Read the model definition and answer for the solid it produces. Units are mm, in the model's axes. Face numbers are marked on the shaded views. A direction names the side the tool comes from. Round coordinates to 2 decimals unless told otherwise and drop trailing zeros. Order: outer loops, then holes, each group sorted by start corner. A loop starts at its lowest first (then second) coordinate and runs counter-clockwise, first axis right, second up. Notation, with made-up numbers: (-21.75, 81.5) - (-13.75, 81.5) arc R8 cw to (-13.75, 95.5) - close; hole circle Ø2 at (-34.75, 36). An arc over 180 degrees is marked (long way). Answer as a JSON object with one key per item and string values. Group by question number.
Q1. A tool of negligible diameter and unlimited length cuts with its end or side. For the marked faces 4, 5 and 6, from which of +Z, -Z, +X, -X, +Y, -Y can it reach the whole face along a straight path? Write none if from no direction.
Q2. A cutting plane is placed at B-B on x = 2.54. Determine the outline of the cut face in (y, z).
Q3. Consider line 1 (X direction, y = -1.25, z = 2.75); line 2 (X direction, y = 8, z = 3.5); line 3 (X direction, y = 0, z = 2). Determine where each line is inside the solid, lowest interval first.
Q4. The mould has two halves that part along Y. Classify the marked faces 1, 2 and 3: pulls with the +Y half, pulls with the -Y half, needs draft (parallel to the pull), parting line crosses it, or undercut.
Q5. A cutting plane is placed at A-A on y = 0. Count the separate pieces of the cut face and the enclosed holes in it, and give its area (3 significant figures).
Q6. Given pin 1 Ø8 at (x, y) = (2.5, -10) entering from +Z; pin 2 Ø2 at (y, z) = (7, 1.5) entering from -X; pin 3 Ø2 at (x, z) = (-10.5, 6) entering from +Y, each flat-ended and moving along its own axis, determine where each tip first touches the part or whether it passes through.
Autodesk Inventor part; units mm, degrees
ref_plane "YZ Plane" through (0, 0, 0) normal (1, 0, 0) x (0, 1, 0)
ref_plane "XZ Plane" through (0, 0, 0) normal (0, 1, 0) x (-1, 0, 0)
ref_plane "XY Plane" through (0, 0, 0) normal (0, 0, 1) x (1, 0, 0)
sketch "Sketch1" plane through (0, 0, 0) normal (0, 0, 1) x (1, 0, 0)
  line L0 (0, 17.78) -> (0, -17.78)
  line L1 (-26.67, 0) -> (26.67, 0)
  line L2 (19.05, -12.7) -> (-19.05, -12.7)
  line L3 (-19.05, -12.7) -> (-19.05, 12.7)
  line L4 (-19.05, 12.7) -> (19.05, 12.7)
  line L5 (19.05, 12.7) -> (19.05, -12.7)
  line L6 (19.05, -12.7) -> (-19.05, 12.7) construction
  line L7 (-19.05, -12.7) -> (19.05, 12.7) construction
  point P0 (0, 0)
  dimension "d0" = 25.4
  dimension "d1" = 38.1
extrude "Extrusion1" add sketch "Sketch1" along normal blind 6.35
sketch "Sketch2" plane through (0, 0, 0) normal (0, 0, 1) x (1, 0, 0)
  line L0 (0, 4.445) -> (0, -4.445)
  line L1 (-14.986, 0) -> (5.461, 0)
  point P0 (0, 0)
  point P1 (2.54, 0)
  point P2 (-12.065, -3.175)
  dimension "d27" = 12.065
  dimension "d35" = 2.54
  dimension "d48" = 3.175
  dimension "d54" = 0
hole "Hole1" at (2.54, 0, 0) direction (0, 0, 1) diameter 4.1402 end through all
sketch "Sketch4" plane through (-19.05, 12.7, 6.35) normal (0, 1, 0) x (1, 0, 0)
  line L0 (19.05, 15.24) -> (19.05, -2.54)
  line L1 (45.72, 6.35) -> (-7.62, 6.35)
  line L2 (38.1, 6.35) -> (38.1, 0)
  line L3 (38.1, 0) -> (0, 0)
  point P0 (19.05, 6.35)
  point P1 (34.29, 3.175)
  point P2 (38.1, 12.7)
  dimension "d36" = 3.81
  dimension "d37" = 3.175
hole "Hole2" at (15.24, 12.7, 3.175) direction (0, -1, 0) diameter 3.175 end through all
hole "Hole3" at (-12.065, -3.175, 0) direction (0, 0, 1) diameter 8.636 end through all counterbore diameter 9.525 counterbore depth 0.635
sketch "Sketch5" plane through (0, 0, 6.35) normal (0, 0, 1) x (1, 0, 0)
  line L0 (19.05, -12.7) -> (19.05, 12.7)
  line L1 (19.05, 12.7) -> (-19.05, 12.7)
  line L2 (-19.05, -12.7) -> (19.05, -12.7)
  line L3 (19.05, 12.7) -> (12.065, 12.7)
  line L4 (12.065, 12.7) -> (12.065, -12.7)
  line L5 (12.065, -12.7) -> (19.05, -12.7)
  line L6 (19.05, -12.7) -> (19.05, 12.7)
  circle A0 centre (2.54, 0) radius 2.0701
  point P0 (0, 0)
  dimension "d39" = 6.985
  dimension "d40" = 9.525
extrude "Extrusion3" add sketch "Sketch5" along normal blind 1.27 contours L2 L4 L1 L0
sketch "Sketch6" plane through (0, 0, 0) normal (0, 0, 1) x (1, 0, 0)
  line L0 (0, 13.335) -> (0, -13.335)
  line L1 (-26.67, 0) -> (26.67, 0)
  line L2 (12.065, 12.7) -> (-19.05, 12.7)
  line L3 (-19.05, -12.7) -> (12.065, -12.7)
  line L4 (19.05, -12.7) -> (19.05, 12.7)
  line L5 (19.05, 12.7) -> (10.16, 12.7)
  line L6 (10.16, 12.7) -> (10.16, 10.0838)
  line L7 (10.16, 10.0838) -> (19.05, 10.0838)
  line L8 (19.05, 10.0838) -> (19.05, 12.7)
  line L9 (19.05, -12.7) -> (10.16, -12.7)
  line L10 (10.16, -12.7) -> (10.16, -10.0838)
  line L11 (10.16, -10.0838) -> (19.05, -10.0838)
  line L12 (19.05, -10.0838) -> (19.05, -12.7)
  point P0 (0, 0)
  dimension "d43" = 2.6162
  dimension "d44" = 2.6162
  dimension "d45" = 8.89
extrude "Extrusion4" cut sketch "Sketch6" along normal up to next contours L2 L5 L4 L7 L6 | L10 L11 L4 L9 L3
sketch "Sketch7" plane through (0, 0, 6.35) normal (0, 0, 1) x (1, 0, 0)
  line L0 (-19.05, 12.7) -> (-19.05, -12.7)
  line L1 (10.16, 12.7) -> (-19.05, 12.7)
  line L2 (-19.05, 12.7) -> (-7.62, 12.7)
  line L3 (-7.62, 12.7) -> (-7.62, 3.175)
  line L4 (-7.62, 3.175) -> (-19.05, 3.175)
  line L5 (-19.05, 3.175) -> (-19.05, 12.7)
  point P0 (0, 0)
  dimension "d49" = 9.525
  dimension "d50" = 11.43
extrude "Extrusion5" cut sketch "Sketch7" against normal up to next
fillet "Fillet2" radius 3.175 1 edges at (-7.62, 3.175, 3.175)
chamfer "Chamfer1" distance 2.54 angle 45 1 edges at (-19.05, 3.175, 3.175)
chamfer "Chamfer2" distance 2.54 angle 45 1 edges at (-19.05, -12.7, 3.175)
chamfer "Chamfer3" distance 3.175 angle 45 1 edges at (12.065, 10.0838, 6.985)
fillet "Fillet3" radius 3.175 1 edges at (-7.62, 12.7, 3.175)
sketch "Sketch8" plane through (0, 0, 6.35) normal (0, 0, 1) x (1, 0, 0)
  line L0 (0, 17.78) -> (0, -17.78)
  line L1 (-26.67, 0) -> (26.67, 0)
  point P0 (0, 0)
  point P1 (-2.54, 6.985)
  point P2 (-2.54, -6.985)
  dimension "d69" = 13.97
  dimension "d70" = 6.985
  dimension "d71" = 2.54
hole "Hole4" at (-2.54, -6.985, 6.35) at (-2.54, 6.985, 6.35) direction (0, 0, -1) diameter 6.35 end through all
sketch "Sketch9" plane through (0, 0, 6.35) normal (0, 0, 1) x (1, 0, 0)
  circle A0 centre (-2.54, 6.985) radius 3.175
  circle A1 centre (-2.54, -6.985) radius 3.175
  line L0 (-1.651, 1.778) -> (-3.429, 1.778)
  line L1 (-3.429, 1.778) -> (-3.429, 12.192)
  line L2 (-3.429, 12.192) -> (-1.651, 12.192)
  line L3 (-1.651, 12.192) -> (-1.651, 1.778)
  line L4 (-1.651, 1.778) -> (-3.429, 12.192) construction
  line L5 (-3.429, 1.778) -> (-1.651, 12.192) construction
  line L6 (-1.651, -12.192) -> (-3.429, -12.192)
  line L7 (-3.429, -12.192) -> (-3.429, -1.778)
  line L8 (-3.429, -1.778) -> (-1.651, -1.778)
  line L9 (-1.651, -1.778) -> (-1.651, -12.192)
  line L10 (-1.651, -12.192) -> (-3.429, -1.778) construction
  line L11 (-3.429, -12.192) -> (-1.651, -1.778) construction
  point P0 (0, 0)
  dimension "d79" = 10.414
  dimension "d80" = 1.778
  dimension "d81" = 10.414
  dimension "d82" = 1.778
extrude "Extrusion6" cut sketch "Sketch9" against normal blind 2.54 contours L3 A0 L1 | A0 L1 L2 L3 | L3 L0 L1 A0 | L9 A1 L7 | A1 L7 L8 L9 | L9 L6 L7 A1
fillet "Fillet4" radius 0.7937 8 edges at (-1.651, -12.192, 5.08) (-3.429, -12.192, 5.08) (-1.651, -1.778, 5.08) (-3.429, -1.778, 5.08) (-1.651, 1.778, 5.08) (-3.429, 1.778, 5.08) (-1.651, 12.192, 5.08) (-3.429, 12.192, 5.08)
chamfer "Chamfer4" distance 1.27 angle 45 1 edges at (-19.05, -4.7625, 0)
chamfer "Chamfer5" distance 0.889 angle 45 2 edges at (-2.54, -3.81, 0) (-2.54, 10.16, 0)
chamfer "Chamfer6" distance 0.127 angle 45 2 edges at (15.24, -10.0838, 1.5875) (15.24, 10.0838, 1.5875)
equation "\"d44\" = d43"
properties part number "J005822" material "ALUMINUM, 6061-T651"
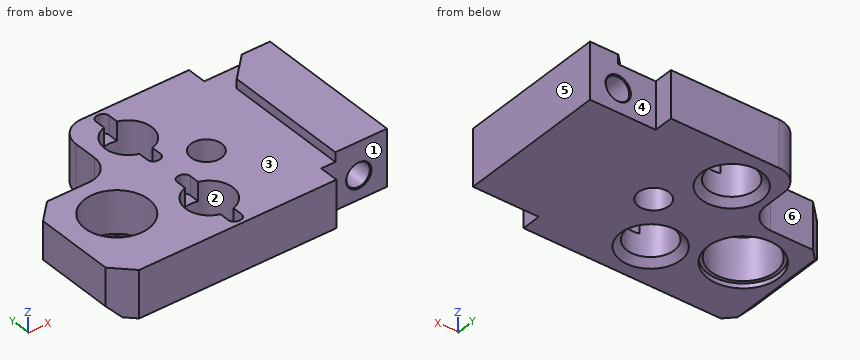
Result set:
{
 "1": {"face 4": "+Z, -Z, +X, +Y", "face 5": "+Z, -Z, +X, +Y, -Y", "face 6": "+Z, -Z, -X, +Y"},
 "2": {"outline": "(-12.7, 0) - (-2.07, 0) - (-2.07, 6.35) - (-12.7, 6.35) - close; (2.07, 0) - (12.7, 0) - (12.7, 6.35) - (2.07, 6.35) - close"},
 "3": {"line 1": "x = -19.05 to -15.93, -8.2 to 0.89, 4.19 to 13.71, 16.77 to 19.05", "line 2": "x = -7.62 to -5.55, 0.47 to 13.69, 16.79 to 19.05", "line 3": "x = -19.05 to -14.99, -9.14 to 0.47, 4.61 to 14.17, 16.31 to 19.05"},
 "4": {"face 1": "pulls with the -Y half", "face 2": "undercut", "face 3": "needs draft"},
 "5": {"separate pieces": "3", "enclosed holes": "1", "area": "178 mm²"},
 "6": {"pin 1": "stops at z = 6.35", "pin 2": "stops at x = -7.64", "pin 3": "stops at y = 3.45"}
}
